For this review, take the finished solid that the model builds, in its own axes (mm). A direction names the side the tool comes from. Give positions to 0.01 mm unless a question says otherwise; leave off trailing zeros. Write each loop counter-clockwise with the first axis right and the second up, starting at its lowest first coordinate (ties: lowest second). Pieces come first, ordered by that corner, then holes. Notation, with made-up numbers: M 62,76.5 L 66,76.5 A14 cw 66,90.5 Z; hole C -36,-23.75 d2. An arc over 180 degrees is marked long. Answer as a JSON object with one key per item and string values. Group by question number.
```python
from build123d import *

# Parameters (mm, degrees)
SKETCH1_W           = 22.3
SKETCH1_H           = 20.2
SKETCH1_R           = 1.65
BOSS_EXTRUDE1_DEPTH = 3.3
SKETCH2_R           = 8.125
BOSS_EXTRUDE2_DEPTH = 12
SKETCH2_3_R         = 1
CUT_EXTRUDE1_DEPTH  = 12


with BuildPart() as part:
    # Sketch1 → Boss-Extrude1 (new body)
    with BuildSketch(Plane.XY):
        with Locations((11.15, 10.1)):
            Rectangle(SKETCH1_W, SKETCH1_H)
        with Locations((2.45, 18)):
            Circle(SKETCH1_R, mode=Mode.SUBTRACT)
        with Locations((19.85, 4.6)):
            Circle(SKETCH1_R, mode=Mode.SUBTRACT)
    extrude(amount=BOSS_EXTRUDE1_DEPTH)

    # Sketch2 → Boss-Extrude2 (add)
    with BuildSketch(Plane.XY.offset(3.3)):
        with Locations((11.15, 11.3)):
            Circle(SKETCH2_R)
    extrude(amount=BOSS_EXTRUDE2_DEPTH)

    # Sketch2<3> → Cut-Extrude1 (cut)
    with BuildSketch(Plane.XY.offset(3.3)):
        with Locations((4.353511594, 1.574306631)):
            Circle(SKETCH2_3_R)
        with Locations((7.380273739, 1.574306631)):
            Circle(SKETCH2_3_R)
        with Locations((10.237837999, 1.574306631)):
            Circle(SKETCH2_3_R)
        with Locations((12.963803906, 1.574306631)):
            Circle(SKETCH2_3_R)
        with Locations((15.708569577, 1.574306631)):
            Circle(SKETCH2_3_R)
        with Locations((18.378136189, 1.574306631)):
            Circle(SKETCH2_3_R)
    extrude(amount=-CUT_EXTRUDE1_DEPTH, mode=Mode.SUBTRACT)


solid = part.part
```
Item 1: Consider section B-B (y = 18.75). Give the boundary of the cut face in (x, z).
Item 2: Consider section C-C (y = 11.3). Give the boundary of the cut face in (x, z) (3 decimals), plus the area to 3 significant figures.
Item 3: Consider section A-A (x = 12.25). Give the boundary of the cut face in (y, z).
Item 4: To check wall thickness, follow probe 1 along Z at (x, y) = (21, 6); probe 2 along Y at (x, z) = (19.85, 1.3); probe 3 along Y at (x, z) = (18, 5.75). State the ranges of each line that lie inside material, in increasing order.
Item 5: Draft analysis for pull direction X (two halves, no side actions). For faces 3 (the flat face through (11, 10, 0)), 4 (the flat face through (0, 10, 2)), 5 (the cylindrical face through (18.2, 4.67, 1.63)), state which applies: released by +X, released by -X, zero draft, split by the parting line, or undercut.
Item 6: Insertion check: P1, Ø8, axis at y = 16.5, z = 12.5, coming from the +X side; P2, Ø3, axis at x = 12.96, y = 1.57, coming from the +Z side; P3, Ø2.5, axis at x = 19.85, y = 4.6, coming from the +Z side; P4, Ø4, axis at x = 2.45, y = 18, coming from the -Z side. Each pin has a flat end and moves straight along its axis. Give the tip position at first contact, or say it passes through.
Item 7: Consider section D-D (z = 1). State how many separate pieces and enclosed holes the cut face has, plus the area to 3 significant figures.
Item 8: Machinability: for faces 1 (the flat face through (3.56, 8, 3.3)), 2 (the flat face through (11, 20.2, 2)), which of the approach directions +Z, -Z, +X, -X, +Y, -Y give a long, thin tool a straight path to every point of the face, cutting with its end or side? Answer none if there is none.
Result set:
{
 "1": {"outline": "M 0,0 L 0.98,0 L 0.98,3.3 L 0,3.3 Z; M 3.92,0 L 22.3,0 L 22.3,3.3 L 14.39,3.3 L 14.39,15.3 L 7.91,15.3 L 7.91,3.3 L 3.92,3.3 Z"},
 "2": {"outline": "M 0,0 L 22.3,0 L 22.3,3.3 L 19.275,3.3 L 19.275,15.3 L 3.025,15.3 L 3.025,3.3 L 0,3.3 Z", "area": "269 mm^2"},
 "3": {"outline": "M 0,0 L 0.87,0 L 0.87,3.3 L 0,3.3 Z; M 2.27,0 L 20.2,0 L 20.2,3.3 L 19.35,3.3 L 19.35,15.3 L 3.25,15.3 L 3.25,3.3 L 2.27,3.3 Z"},
 "4": {"probe 1": "z = 0 to 3.3", "probe 2": "y = 0 to 2.95, 6.25 to 20.2", "probe 3": "y = 6.93 to 15.67"},
 "5": {"face 3": "zero draft", "face 4": "released by -X", "face 5": "undercut"},
 "6": {"P1": "stops at x = 19.19", "P2": "stops at z = 3.3", "P3": "passes through", "P4": "stops at z = 0"},
 "7": {"separate pieces": "1", "enclosed holes": "8", "area": "415 mm^2"},
 "8": {"face 1": "+Z", "face 2": "+Z, -Z, +X, -X, +Y"}
}
